Here's the drawing with two shaded views (mm, measured from the low corner). I have some questions. Round coordinates to 2 decimals unless told otherwise and drop trailing zeros. Order: outer loops, then holes, each group sorted by start corner. A loop starts at its lowest first (then second) coordinate and runs counter-clockwise, first axis right, second up.
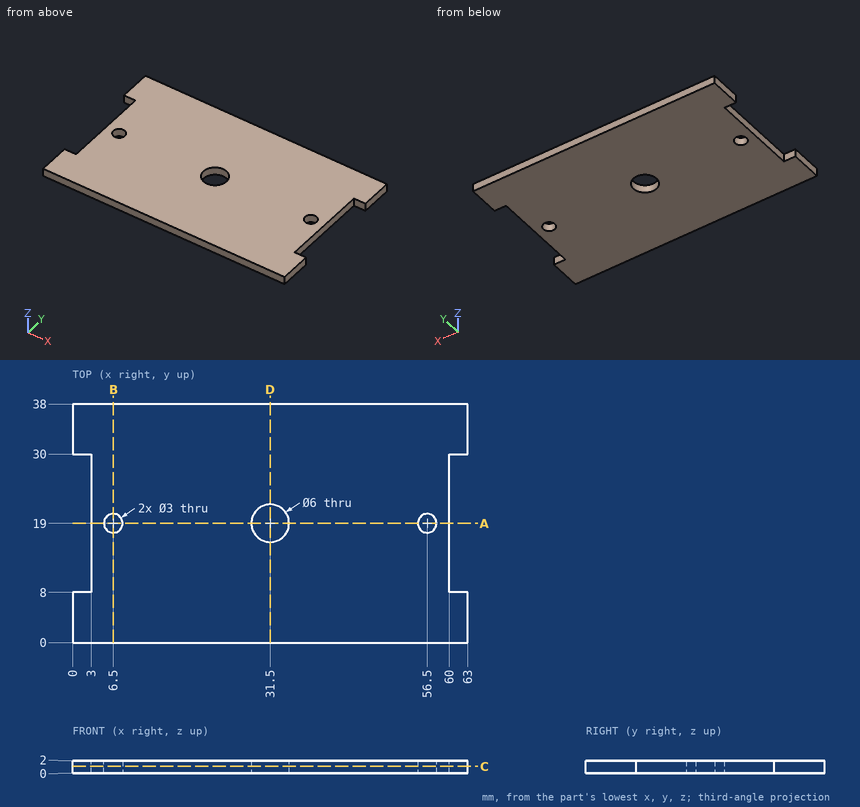
1. I'm going to push flat-ended pins straight in: P1, Ø0.6, axis at y = 14, z = 1.5, coming from the +X side; P2, Ø12, axis at x = 42, y = 20, coming from the -Z side; P3, Ø1, axis at y = 16.5, z = 0.5, coming from the -X side. Where does each tip first touch, or does it pass through?
Evaluation:
P1: stops at x = 60
P2: stops at z = 0
P3: stops at x = 3
2. I need wall thicknesses on probe 1 along Y at (x, z) = (6.5, 1.2); probe 2 along X at (y, z) = (20, 0.95); probe 3 along X at (y, z) = (14, 1). Which ranges of each line are inside material? Lowest first, please.
Evaluation:
probe 1: y = 0 to 17.5, 20.5 to 38
probe 2: x = 3 to 5.38, 7.62 to 28.67, 34.33 to 55.38, 57.62 to 60
probe 3: x = 3 to 60
3. If we section it at A-A, the plane y = 19: Write out the boundary of the cut face in (x, z), and give its area (3 significant figures).
Evaluation:
outline: (3, 0) - (5, 0) - (5, 2) - (3, 2) - close; (8, 0) - (28.5, 0) - (28.5, 2) - (8, 2) - close; (34.5, 0) - (55, 0) - (55, 2) - (34.5, 2) - close; (58, 0) - (60, 0) - (60, 2) - (58, 2) - close
area: 90.0 mm2
4. If we section it at D-D, the plane x = 31.5: Write out the boundary of the cut face in (y, z).
Evaluation:
outline: (0, 0) - (16, 0) - (16, 2) - (0, 2) - close; (22, 0) - (38, 0) - (38, 2) - (22, 2) - close
5. If we section it at C-C, the plane z = 1.05: Write out the boundary of the cut face in (x, y).
Evaluation:
outline: (0, 0) - (63, 0) - (63, 8) - (60, 8) - (60, 30) - (63, 30) - (63, 38) - (0, 38) - (0, 30) - (3, 30) - (3, 8) - (0, 8) - close; hole circle Ø3 at (6.5, 19); hole circle Ø6 at (31.5, 19); hole circle Ø3 at (56.5, 19)
6. If we section it at B-B, the plane x = 6.5: Write out the boundary of the cut face in (y, z), and give its area (3 significant figures).
Evaluation:
outline: (0, 0) - (17.5, 0) - (17.5, 2) - (0, 2) - close; (20.5, 0) - (38, 0) - (38, 2) - (20.5, 2) - close
area: 70.0 mm2
